Check sheet for the modelled part. Datum: model origin and axes. Units: mm. Face numbers are marked on the shaded views. A direction names the side the tool comes from. Round coordinates to 2 decimals unless told otherwise and drop trailing zeros. Write each loop counter-clockwise with the first axis right and the second up, starting at its lowest first coordinate (ties: lowest second). Pieces come first, ordered by that corner, then holes. Notation, with made-up numbers: M 0.25,37.25 L 33.25,37.25 A25 ccw 33.25,54.25 Z; hole C 27,52 d6. An arc over 180 degrees is marked long. One line per item, written item: value.
from build123d import *

# Parameters (mm, degrees)
SKETCH1_W           = 10.16
SKETCH1_H           = 5.08
SKETCH1_R           = 6.049999965
BOSS_EXTRUDE1_DEPTH = 25.4
SKETCH6_W           = 11.43
SKETCH6_H           = 25.4
BOSS_EXTRUDE3_DEPTH = 50.8
CHAMFER2_DEPTH      = 25.4
SKETCH4_R           = 2.032
CUT_EXTRUDE2_DEPTH  = 12.7


with BuildPart() as part:
    # Sketch1 → Boss-Extrude1 (new body)
    # profile 1 of 4: a face of its own
    with BuildSketch(Plane(origin=(0, 0, 0), x_dir=(1, 0, 0), z_dir=(0, 1, 0))):
        with BuildLine():
            Line((-5.08, -8.057246738), (-5.08, -14.407246738))
            Line((-5.08, -14.407246738), (5.08, -14.407246738))
            Line((5.08, -14.407246738), (5.08, -8.057246738))
            ThreePointArc((5.08, -8.057246738), (0, -9.525), (-5.08, -8.057246738))
        make_face()
    # profile 2 of 4: a face of its own
    with BuildSketch(Plane(origin=(0, 0, 0), x_dir=(1, 0, 0), z_dir=(0, 1, 0))):
        with Locations((0, -16.947246738)):
            Rectangle(SKETCH1_W, SKETCH1_H)
    # profile 3 of 4: a face of its own
    with BuildSketch(Plane(origin=(0, 0, 0), x_dir=(1, 0, 0), z_dir=(0, 1, 0))):
        with BuildLine():
            ThreePointArc((9.525, 0), (-4.601012117, 8.340042716), (-5.08, -8.057246738))
            Line((-5.08, -8.057246738), (5.08, -8.057246738))
            ThreePointArc((5.08, -8.057246738), (8.340042716, -4.601012117), (9.525, 0))
        make_face()
        with Locations(Location((0, 0, 0), (0, 0, 270))):
            Circle(SKETCH1_R, mode=Mode.SUBTRACT)
    # profile 4 of 4: a face of its own
    with BuildSketch(Plane(origin=(0, 0, 0), x_dir=(1, 0, 0), z_dir=(0, 1, 0))):
        with BuildLine():
            Line((5.08, -8.057246738), (-5.08, -8.057246738))
            ThreePointArc((-5.08, -8.057246738), (0, -9.525), (5.08, -8.057246738))
        make_face()
    extrude(amount=BOSS_EXTRUDE1_DEPTH)

    # Sketch6 → Boss-Extrude3 (add)
    with BuildSketch(Plane.ZY.offset(5.08)):
        with Locations((13.772246738, 12.7)):
            Rectangle(SKETCH6_W, SKETCH6_H)
    extrude(amount=BOSS_EXTRUDE3_DEPTH)

    # Chamfer2: read off the stored shape, not the designer's step
    # Chamfer2 outline → Chamfer2 (add)
    with BuildSketch(Plane(origin=(0, 0, 0), x_dir=(1, 0, 0), z_dir=(0, 1, 0))):
        with BuildLine():
            Line((-5.261303905, 7.940044472), (-55.88, -7.308719642))
            Line((-55.88, -7.308719642), (-55.88, -8.057246738))
            Line((-55.88, -8.057246738), (-5.08, -8.057246738))
            ThreePointArc((-5.08, -8.057246738), (-9.524388334, -0.107943825), (-5.261303905, 7.940044472))
        make_face()
    extrude(amount=CHAMFER2_DEPTH)

    # Sketch4 → Cut-Extrude2 (cut)
    with BuildSketch(Plane.XY.offset(19.487246738)):
        with Locations((0, 19.05)):
            Circle(SKETCH4_R)
        with Locations((0, 6.35)):
            Circle(SKETCH4_R)
        with Locations((-50.8, 19.05)):
            Circle(SKETCH4_R)
        with Locations((-50.8, 6.35)):
            Circle(SKETCH4_R)
    extrude(amount=-CUT_EXTRUDE2_DEPTH, mode=Mode.SUBTRACT)


solid = part.part
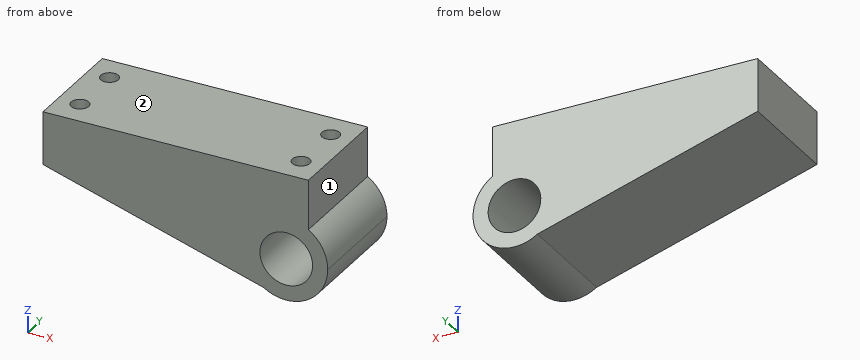
Q1. Sectioned sample at B-B on y = 6.35. Enter the section's corners in (x, z) (3 decimals).
Completed:
outline: M -55.88,7.309 L -5.261,-7.94 A9.525 ccw long 5.08,8.057 L 5.08,19.487 L 2.032,19.487 L 2.032,6.787 L -2.032,6.787 L -2.032,19.487 L -48.768,19.487 L -48.768,6.787 L -52.832,6.787 L -52.832,19.487 L -55.88,19.487 Z; hole C 0,0 d12.1
Q2. Scan lines: line 1 (Y direction, x = -50.8, z = 10.25); line 2 (X direction, y = 23.5, z = 12.5); line 3 (Z direction, x = -20.5, y = 22.5). Record each from-to range of solid material in increasing order. Write a range as [from, to].
Completed:
line 1: [0, 4.32], [8.38, 17.02], [21.08, 25.4]
line 2: [-55.88, 5.08]
line 3: [-3.35, 19.49]
Q3. Sectioned sample at D-D on y = 3.5. Enter the section's corners in (x, z) (3 decimals), and give its area (3 significant figures).
Completed:
outline: M -55.88,7.309 L -5.261,-7.94 A9.525 ccw long 5.08,8.057 L 5.08,19.487 L -55.88,19.487 Z; hole C 0,0 d12.1
area: 1,230 mm^2
Q4. Sectioned sample at A-A on x = 0. Enter the section's corners in (y, z) (3 decimals).
Completed:
outline: M 0,-9.525 L 25.4,-9.525 L 25.4,-6.05 L 0,-6.05 Z; M 0,6.05 L 25.4,6.05 L 25.4,19.487 L 21.082,19.487 L 21.082,6.787 L 17.018,6.787 L 17.018,19.487 L 8.382,19.487 L 8.382,6.787 L 4.318,6.787 L 4.318,19.487 L 0,19.487 Z
Q5. Depth check by flat-ended pin: P1, Ø3, axis at x = -11, y = 16, coming from the -Z side; P2, Ø2.5, axis at x = -50.8, y = 6.35, coming from the -Z side; P3, Ø1.2, axis at x = -51, y = 18.5, coming from the +Z side. Enter the tip coordinate at first touch or a pass-through.
Completed:
P1: z = -6.66
P2: z = 5.4
P3: z = 6.79
Q6. Sectioned sample at C-C on z = 0.75. Enter the section's corners in (x, y), and give its area (3 significant figures).
Completed:
outline: M -34.11,0 L -6,0 L -6,25.4 L -34.11,25.4 Z; M 6,0 L 9.5,0 L 9.5,25.4 L 6,25.4 Z
area: 803 mm^2
Q7. Access from +Z, -Z, +X, -X, +Y, -Y to the whole of each face (thin tool, end or side, straight path). Record for the marked faces 1 and 2.
Completed:
face 1: +Z, +X, +Y, -Y
face 2: +Z, +X, -X, +Y, -Y
